Geometry: see drawing. Coordinates: mm, zero at the bounding-box minimum. Round coordinates to 2 decimals unless told otherwise and drop trailing zeros. Loops run counter-clockwise (first coordinate to the right, second up) from the corner with the lowest first, then second, coordinate; pieces in that order, holes last. Notation, with made-up numbers: (23.25, 77) - (40.25, 77) arc R14 ccw to (40.25, 98) - close; hole circle Ø2 at (89.25, -5). An arc over 180 degrees is marked (long way). Write item = value, one per line. Start each with the question number.
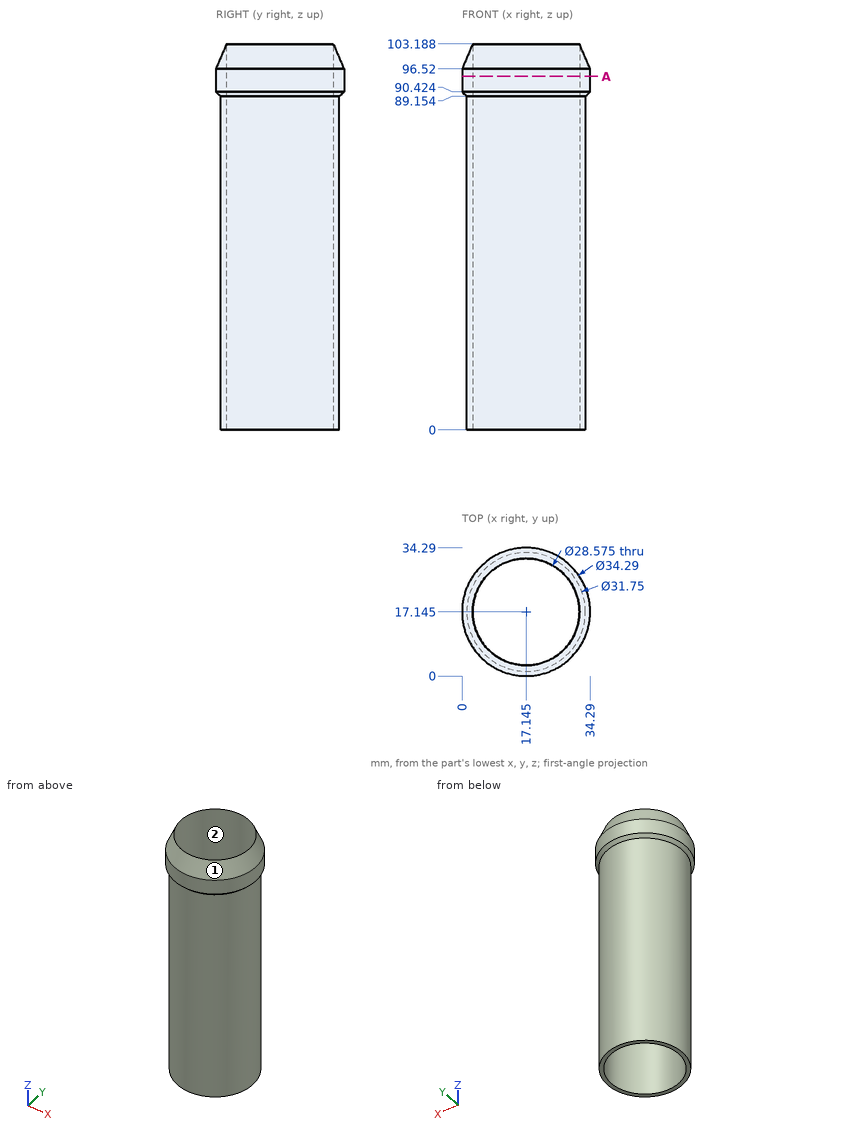
(1) Mould query, pull axis Y, two halves, no side actions, for the marked faces 1 and 2. Classes: +Y half, -Y half, draft (parallel to the pull), parting line (faces both ways), or undercut.
(2) Cut plane A-A (z = 94.5). Output: boundary loops of the cut face in (x, y) (1 decimal), and give its area (3 significant figures).
(3) Material intervals for line 1 along Y through (x, z) = (16.5, 90.5); line 2 along Y through (x, z) = (24.5, 9) (1 decimal); line 3 along X through (y, z) = (17.5, 68.5) (1 decimal), sorted ascending. Write a range as from..to.
(4) Pin query (flat end, axial travel): P1, Ø5, axis at x = 4.5, z = 92.5, coming from the -Y side (1 decimal); P2, Ø1.5, axis at x = 19, z = 15, coming from the -Y side; P3, Ø5, axis at y = 11.5, z = 43.5, coming from the -X side (1 decimal); P4, Ø17, axis at x = 17.145, y = 17.145, coming from the +Z side. Return the tip coordinate at first contact, or that it passes through.
Solution:
q1.face_1 = parting line
q1.face_2 = undercut
q2.outline = circle Ø34.3 at (17.1, 17.1); hole circle Ø28.6 at (17.1, 17.1)
q2.area = 282 mm^2
q3.line_1 = 0.01..2.87, 31.42..34.28
q3.line_2 = 3.1..4.9, 29.4..31.2
q3.line_3 = 1.3..2.9, 31.4..33
q4.P1 = 3.3
q4.P2 = 1.31
q4.P3 = 1.6
q4.P4 = through
